Model file for the job. Use its own axes, mm. A direction names the side the tool comes from. Round coordinates to 2 decimals unless told otherwise and drop trailing zeros. Order: outer loops, then holes, each group sorted by start corner. A loop starts at its lowest first (then second) coordinate and runs counter-clockwise, first axis right, second up. Notation, with made-up numbers: (-27, 68.5) -> (24, 68.5) arc R21 ccw to (24, 91.5) -> close; hole circle Ø2 at (-10, 38). An arc over 180 degrees is marked (long way). Use CSV: the item, a comma, the result in double quotes.
```python
from build123d import *

# Parameters (mm, degrees)
F0_R      = 40
F1_DEPTH  = 76.2
F2_R      = 10.5
F3_DEPTH  = 63.5
F4_W      = 7.348393
F4_H      = 15.5
F5_DEPTH  = 53.34
F7_W      = 15.24
F7_H      = 15
F8_DEPTH  = 15.24
F9_W      = 30
F9_H      = 15
F10_DEPTH = 13


with BuildPart() as f1:
    # F0 (on Top) → F1 (new body)
    with BuildSketch(Plane.XY):
        Circle(F0_R)
    extrude(amount=F1_DEPTH)

    # F2 (on Top) → F3 (cut)
    with BuildSketch(Plane.XY):
        Circle(F2_R)
    extrude(amount=F3_DEPTH, mode=Mode.SUBTRACT)

    # F4 (on Top) → F5 (cut)
    with BuildSketch(Plane.XY):
        with Locations((11.025803, -0.5)):
            Rectangle(F4_W, F4_H)
    extrude(amount=F5_DEPTH, mode=Mode.SUBTRACT)

    # F7 (on offset) → F8 (cut)
    with BuildSketch(Plane.XY.offset(53.5)):
        with Locations((-7.62, 0)):
            Rectangle(F7_W, F7_H)
    extrude(amount=-F8_DEPTH, mode=Mode.SUBTRACT)

    # F9 (on Front) → F10 (cut)
    with BuildSketch(Plane.XZ):
        with Locations((0, 45.916821)):
            Rectangle(F9_W, F9_H)
    extrude(amount=-F10_DEPTH, mode=Mode.SUBTRACT)


solid = f1.part
```
Q1. Which spindle directions (+Z, -Z, +X, -X, +Y, -Y) get a long thin tool onto all of the face, cutting with end or side? Do faces 4 (the flat face through (-15.24, 0, 46)), 5 (the cylindrical face through (-8.33, -6.39, 31.31)), 6 (the flat face through (-1, 1, 76.2)). Say none if no direction does.
From the geometry:
face 4,"none"
face 5,"-Z"
face 6,"+Z, +X, -X, +Y, -Y"
Q2. Cut at D-D (z = 55). Give the cut face in (x, y).
From the geometry:
outline,"circle Ø80 at (0, 0); hole circle Ø21 at (0, 0)"
Q3. Mould opens along X. For faces 1 (the flat face through (-9, -8, 0)), 2 (the flat face through (0, 13, 46)), 3 (the cylindrical face through (-8.67, -39.05, 37.57)) say: +X half, -X half, draft (parallel to the pull), parting line (faces both ways), or undercut.
From the geometry:
face 1,"draft"
face 2,"undercut"
face 3,"parting line"
Q4. Probe line 1 along Y through (x, z) = (0, 45); line 2 along Y through (x, z) = (0, 32); line 3 along Z through (x, y) = (-11, -3.5). List the from-to ranges inside material, lowest first.
From the geometry:
line 1,"y = -40 to -10.5, 13 to 40"
line 2,"y = -40 to -10.5, 10.5 to 40"
line 3,"z = 0 to 38.26, 53.5 to 76.2"
Q5. Cut at B-B (x = 0). Give the cut face in (y, z).
From the geometry:
outline,"(-40, 0) -> (-10.5, 0) -> (-10.5, 63.5) -> (10.5, 63.5) -> (10.5, 53.42) -> (13, 53.42) -> (13, 38.42) -> (10.5, 38.42) -> (10.5, 0) -> (40, 0) -> (40, 76.2) -> (-40, 76.2) -> close"
Q6. Cut at A-A (z = 27.5). Give the cut face in (x, y).
From the geometry:
outline,"circle Ø80 at (0, 0); hole (7.35, -8.25) -> (14.7, -8.25) -> (14.7, 7.25) -> (7.6, 7.25) arc R10.5 ccw (long way) to (7.35, -7.5) -> close"
Q7. Cut at C-C (y = 32). Give the cut face in (x, z), plus the area to 3 significant figures.
From the geometry:
outline,"(-24, 0) -> (24, 0) -> (24, 76.2) -> (-24, 76.2) -> close"
area,"3,660 mm²"
Q8. Pin check, flat tips, straight feed: pin 1 (8.5 mm diameter, centred on x = -11.5, z = 44.5, fed in from +Y); pin 2 (3.5 mm diameter, centred on x = 12.5, z = 36, fed in from +Y); pin 3 (2 mm diameter, centred on y = 13, z = 29.5, fed in from -X). Stop position of each tip, or through.
From the geometry:
pin 1,"stops at y = 39.34"
pin 2,"stops at y = 38.53"
pin 3,"stops at x = -38.16"
